```python
from build123d import *

# Parameters (mm, degrees)
F0_R     = 12.5
F1_DEPTH = 10
F2_SIZE  = 3
F3_R     = 5.25
F4_DEPTH = 8


# Not quite as in the source:
# - a feature names something its author has since deleted; it is built from what else it names


with BuildPart() as f1:
    # F0 (on Top) → F1 (new body)
    with BuildSketch(Plane.XY):
        Circle(F0_R)
    extrude(amount=F1_DEPTH)

    # F2
    f2_edges = [f1.edges().sort_by_distance(p)[0] for p in [
        (-12.5, 0, 10),
        (12.5, 0, 5),
        (-12.5, 0, 0),
    ]]
    chamfer(f2_edges, length=F2_SIZE)

    # F3 (on face) → F4 (cut)
    with BuildSketch(Plane(origin=(0, 0, 0), x_dir=(1, 0, 0), z_dir=(0, 0, -1))):
        Circle(F3_R)
    extrude(amount=-F4_DEPTH, mode=Mode.SUBTRACT)


solid = f1.part
```
The model under review builds one solid part; all positions refer to its coordinate system, in mm. A direction names the side the tool comes from. Give positions to 0.01 mm unless a question says otherwise; leave off trailing zeros. Order: outer loops, then holes, each group sorted by start corner. A loop starts at its lowest first (then second) coordinate and runs counter-clockwise, first axis right, second up. Notation, with made-up numbers: (3, 0) - (36, 0) arc R14 ccw to (36, 25) - close; hole circle Ø5 at (42.25, 9.25). An arc over 180 degrees is marked (long way). Use CSV: the item, a comma, the result in double quotes. Start each with the question number.
Q1. To check wall thickness, follow line 1 along Y through (x, z) = (0, 5.5); line 2 along X through (y, z) = (-2.5, 4); line 3 along Z through (x, y) = (-1, 1.5). State the ranges of each line that lie inside material, in increasing order. Write a range as [from, to].
Q2. We need section A-A, the plane y = 0. Write out the cut boundary in (x, z).
Q3. The part is to be moulded in two halves that separate along X. For faces 1 (the cylindrical face through (5, -1.6, 3.9)), 2 (the cylindrical face through (11.923, 3.755, 4.972)), 3 (the flat face through (0, 0, 10)), say which applies: +X half, -X half, draft (parallel to the pull), parting line (faces both ways), or undercut.
Q4. Clearance check with flat-ended pins moving along their axes: pin 1 Ø6 at (y, z) = (-5.5, 8.5) entering from -X; pin 2 Ø6 at (x, z) = (-3.5, 3) entering from -Y; pin 3 Ø4 at (y, z) = (6.5, 2.5) entering from +X; pin 4 Ø12 at (x, y) = (1.5, 8.5) entering from -Z. State where each tip first meets the part, or that it passes through.
Q5. Tool access review of faces 4 (the conical face through (-2.09, -9.42, 9.85)), 5 (the flat face through (0, 0, 8)): name each direction out of +Z, -Z, +X, -X, +Y, -Y from which nothing blocks a thin tool from reaching the whole face with its end or side.
Q6. We need section C-C, the plane z = 1.25. Write out the cut boundary in (x, y), and give its area (3 significant figures).
Outcome:
1,line 1,"y = [-12.5, -5.25], [5.25, 12.5]"
1,line 2,"x = [-12.25, -4.62], [4.62, 12.25]"
1,line 3,"z = [8, 10]"
2,outline,"(-12.5, 3) - (-9.5, 0) - (-5.25, 0) - (-5.25, 8) - (5.25, 8) - (5.25, 0) - (9.5, 0) - (12.5, 3) - (12.5, 7) - (9.5, 10) - (-9.5, 10) - (-12.5, 7) - close"
3,face 1,"undercut"
3,face 2,"parting line"
3,face 3,"draft"
4,pin 1,"stops at x = -12.16"
4,pin 2,"stops at y = -12.49"
4,pin 3,"stops at x = 11.64"
4,pin 4,"stops at z = 0"
5,face 4,"+Z"
5,face 5,"-Z"
6,outline,"circle Ø21.5 at (0, 0); hole circle Ø10.5 at (0, 0)"
6,area,"276 mm^2"
